Part model, mm, in its own coordinate system. Coordinates: 2 decimals unless noted, no trailing zeros. Loops run counter-clockwise (first coordinate to the right, second up) from the corner with the lowest first, then second, coordinate; pieces in that order, holes last. Notation, with made-up numbers: (44, -25.5) - (79, -25.5) arc R22 cw to (79, -17.5) - close; hole circle Ø8 at (3, 55.5). An arc over 180 degrees is marked (long way). Use a Markdown table: item, result. Add a question column.
1. Wall check: probe 1 along X at (y, z) = (0.2, 0); probe 2 along Y at (x, z) = (20.5, 3); probe 3 along Z at (x, y) = (-9, 0.05). Give the ranges that are in metal, low to high. Write a range as [from, to].
2. Band-saw the part on D-D, the plane x = 19. Give the cut face in (y, z), plus the area to 3 significant figures.
3. Band-saw the part on B-B, the plane x = 3. Give the cut face in (y, z).
4. Drop flat-ended pins along their axis: pin 1 (1 mm diameter, centred on x = -4, y = 0, fed in from +Z); pin 2 (6 mm diameter, centred on x = 10.5, z = 0.5, fed in from -Y); pin 3 (0.6 mm diameter, centred on y = -2, z = -20, fed in from +X); pin 4 (21 mm diameter, centred on x = 0, z = 0, fed in from -Y). Give the stop position or say it passes through.
5. Band-saw the part on A-A, the plane z = 0. Give the cut face in (x, y), plus the area to 3 significant figures.
6. Pull direction Z, two halves, no side cores. Call faces 1 (the flat face through (10, 0, 9)), 2 (the cylindrical face through (-20, -1, 0)), 3 (the flat face through (10, 0.5, 9)), 4 (the cylindrical face through (-19.495, -1.268, -0.429)): pulls with the +Z half, pulls with the -Z half, needs draft (parallel to the pull), parting line crosses it, or undercut.
7. Band-saw the part on C-C, the plane y = -1.35. Give the cut face in (x, z), plus the area to 3 significant figures.
from build123d import *

# Parameters (mm, degrees)
EXTRUDE_1_DEPTH     = 0.5
EXTRUDE_START       = 2.5
EXTRUDE_2_DEPTH     = 2.5
SKETCH_3_R          = 13
CUT_EXTRUDE_1_DEPTH = 30.883105595


with BuildPart() as part:
    # 草图1 → 凸台-拉伸1 (new body)
    with BuildSketch(Plane(origin=(0, 0, 0), x_dir=(1, 0, 0), z_dir=(0, 1, 0))):
        with BuildLine():
            ThreePointArc((20, 0), (14.142135624, 14.142135624), (0, 20))
            Line((0, 20), (0, -20))
            ThreePointArc((0, -20), (14.142135624, -14.142135624), (20, 0))
        make_face()
        with BuildLine():
            Line((0, -20), (0, 20))
            ThreePointArc((0, 20), (-20, 0), (0, -20))
        make_face()
        with BuildLine():
            Line((22, 20), (0, 20))
            ThreePointArc((0, 20), (14.142135624, 14.142135624), (20, 0))
            ThreePointArc((20, 0), (14.142135624, -14.142135624), (0, -20))
            Line((0, -20), (22, -20))
            Line((22, -20), (22, 20))
        make_face()
    extrude(amount=EXTRUDE_1_DEPTH)

    # 草图2 → 凸台-拉伸2 (add)
    with BuildSketch(Plane.XZ.offset(EXTRUDE_START)):
        with BuildLine():
            Line((0, 19.5), (0, 20))
            ThreePointArc((0, 20), (-20, 0), (0, -20))
            Line((0, -20), (0, -19.5))
            ThreePointArc((0, -19.5), (-19.5, 0), (0, 19.5))
        make_face()
    extrude(amount=-EXTRUDE_2_DEPTH)

    # 草图3 → 切除-拉伸1 (cut, through all)
    with BuildSketch(Plane(origin=(0, 0.5, 0), x_dir=(1, 0, 0), z_dir=(0, 1, 0))):
        with Locations(Location((0, 0, 0), (0, 0, 270))):
            Circle(SKETCH_3_R)
    extrude(amount=-CUT_EXTRUDE_1_DEPTH, mode=Mode.SUBTRACT)


solid = part.part
Geometry check:
| question | item | result |
|---|---|---|
| 1 | probe 1 | x = [-20, -13], [13, 22] |
| 1 | probe 2 | y = [0, 0.5] |
| 1 | probe 3 | z = [-17.86, -9.38], [9.38, 17.86] |
| 2 | outline | (0, -20) - (0.5, -20) - (0.5, 20) - (0, 20) - close |
| 2 | area | 20.0 mm^2 |
| 3 | outline | (0, -20) - (0.5, -20) - (0.5, -12.65) - (0, -12.65) - close; (0, 12.65) - (0.5, 12.65) - (0.5, 20) - (0, 20) - close |
| 4 | pin 1 | stops at z = 19.69 |
| 4 | pin 2 | stops at y = 0 |
| 4 | pin 3 | stops at x = 0 |
| 4 | pin 4 | passes through |
| 5 | outline | (-20, -2.5) - (-19.5, -2.5) - (-19.5, 0) - (-13, 0) - (-13, 0.5) - (-20, 0.5) - close; (13, 0) - (22, 0) - (22, 0.5) - (13, 0.5) - close |
| 5 | area | 9.25 mm^2 |
| 6 | face 1 | undercut |
| 6 | face 2 | parting line crosses it |
| 6 | face 3 | needs draft |
| 6 | face 4 | undercut |
| 7 | outline | (0, -20) - (0, -19.5) arc R19.5 cw to (0, 19.5) - (0, 20) arc R20 ccw to start |
| 7 | area | 31.0 mm^2 |
